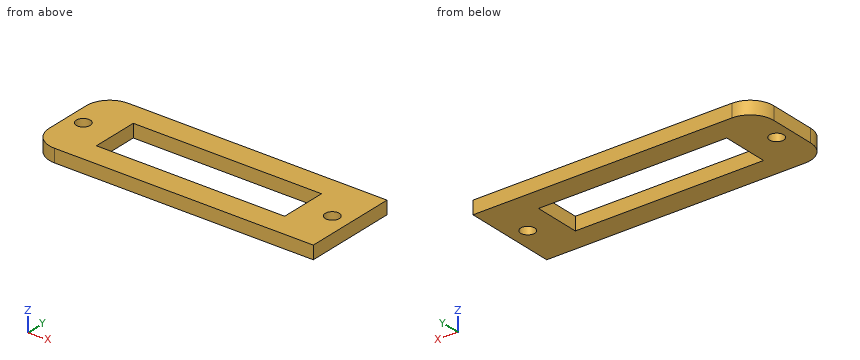
Autodesk Inventor part; units mm, degrees
ref_plane "YZ Plane" through (0, 0, 0) normal (1, 0, 0) x (0, 1, 0)
ref_plane "XZ Plane" through (0, 0, 0) normal (0, 1, 0) x (-1, 0, 0)
ref_plane "XY Plane" through (0, 0, 0) normal (0, 0, 1) x (1, 0, 0)
sketch "Sketch1" plane through (0, 0, 0) normal (0, 0, 1) x (1, 0, 0)
  line L0 (-43.2426, 0) -> (42.2071, 0)
  line L1 (0, -15.4497) -> (0, 15.4497)
  line L2 (-25, 10) -> (30, 10)
  line L3 (30, 10) -> (30, -10)
  line L4 (30, -10) -> (-25, -10)
  line L5 (-30, -5) -> (-30, 5)
  arc A0 (-25, 10) -> (-30, 5) centre (-25, 5) ccw
  arc A1 (-30, -5) -> (-25, -10) centre (-25, -5) ccw
  point P0 (0, 0)
  point P1 (-30, 10)
  point P2 (-30, -10)
  dimension "d0" = 60
  dimension "d1" = 20
  dimension "d2" = 30
  dimension "d3" = 10
  dimension "d6" = 5
extrude "Extrusion1" add sketch "Sketch1" along normal blind 2.8
sketch "Sketch2" plane through (0, 0, 2.8) normal (0, 0, 1) x (1, 0, 0)
  line L0 (30, 10) -> (30, -10)
  line L1 (-30, -5) -> (-30, 5)
  circle A0 centre (-26.7, 0) radius 1.5
  circle A1 centre (26.2, 0) radius 1.5
  line L2 (-25, 10) -> (30, 10)
  line L3 (-20, 5) -> (20, 5)
  line L4 (20, 5) -> (20, -5)
  line L5 (20, -5) -> (-20, -5)
  line L6 (-20, -5) -> (-20, 5)
  point P0 (0, 0)
  dimension "d7" = 3
  dimension "d8" = 3
  dimension "d9" = 3.8
  dimension "d10" = 3.3
  dimension "d13" = 40
  dimension "d14" = 10
  dimension "d15" = 5
  dimension "d16" = 20
extrude "Extrusion2" cut sketch "Sketch2" against normal blind 10
equation "\"d2\" = 0.5 * d0"
equation "\"d3\" = 0.5 * d1"
properties part number "Acrylic_PitchServoSupport_1"
Design review of the part built by this model. Coordinates are the model's own, in mm. Give positions to 0.01 mm unless a question says otherwise; leave off trailing zeros. Write each loop counter-clockwise with the first axis right and the second up, starting at its lowest first coordinate (ties: lowest second). Pieces come first, ordered by that corner, then holes. Notation, with made-up numbers: (74, 48) - (82, 48) arc R20 ccw to (82, 69) - close; hole circle Ø4 at (86, -21.5). An arc over 180 degrees is marked (long way). Return JSON: item names as keys, results as strings. Group by question number.
(1) Insertion check: pin 1 (1.8 mm diameter, centred on x = 26.2, y = 0, fed in from +Z). The pin has a flat end and moves straight along its axis. Give the tip position at first contact, or say it passes through.
(2) We need section B-B, the plane x = 2. Give the boundary of the cut face in (y, z), then the cut area to 3 significant figures.
(3) We need section A-A, the plane y = 4. Give the boundary of the cut face in (x, z).
(4) To check wall thickness, follow probe 1 along Y at (x, z) = (-12, 1.2); probe 2 along X at (y, z) = (-1.25, 0.8); probe 3 along X at (y, z) = (2.25, 0.1). State the ranges of each line that lie inside material, in increasing order.
(5) We need section C-C, the plane y = 0. Give the boundary of the cut face in (x, z), then the cut area to 3 significant figures.
(6) We need section D-D, the plane z = 0.65. Give the boundary of the cut face in (x, y), then the cut area to 3 significant figures.
Reported:
{
 "1": {"pin 1": "passes through"},
 "2": {"outline": "(-10, 0) - (-5, 0) - (-5, 2.8) - (-10, 2.8) - close; (5, 0) - (10, 0) - (10, 2.8) - (5, 2.8) - close", "area": "28.0 mm2"},
 "3": {"outline": "(-30, 0) - (-20, 0) - (-20, 2.8) - (-30, 2.8) - close; (20, 0) - (30, 0) - (30, 2.8) - (20, 2.8) - close"},
 "4": {"probe 1": "y = -10 to -5, 5 to 10", "probe 2": "x = -30 to -27.53, -25.87 to -20, 20 to 25.37, 27.03 to 30", "probe 3": "x = -30 to -20, 20 to 30"},
 "5": {"outline": "(-30, 0) - (-28.2, 0) - (-28.2, 2.8) - (-30, 2.8) - close; (-25.2, 0) - (-20, 0) - (-20, 2.8) - (-25.2, 2.8) - close; (20, 0) - (24.7, 0) - (24.7, 2.8) - (20, 2.8) - close; (27.7, 0) - (30, 0) - (30, 2.8) - (27.7, 2.8) - close", "area": "39.2 mm2"},
 "6": {"outline": "(-30, -5) arc R5 ccw to (-25, -10) - (30, -10) - (30, 10) - (-25, 10) arc R5 ccw to (-30, 5) - close; hole circle Ø3 at (-26.7, 0); hole (-20, -5) - (20, -5) - (20, 5) - (-20, 5) - close; hole circle Ø3 at (26.2, 0)", "area": "775 mm2"}
}
